Could you check a few things on this model? Use its own coordinates, in mm. Give positions to 0.01 mm unless a question says otherwise; leave off trailing zeros. Write each loop counter-clockwise with the first axis right and the second up, starting at its lowest first coordinate (ties: lowest second). Pieces come first, ordered by that corner, then holes. Notation, with made-up numbers: M 65.5,30.25 L 115.5,30.25 A14 cw 115.5,34.25 Z; hole C -3.5,69.25 d9. An arc over 180 degrees is marked long. One line per item, written item: value.
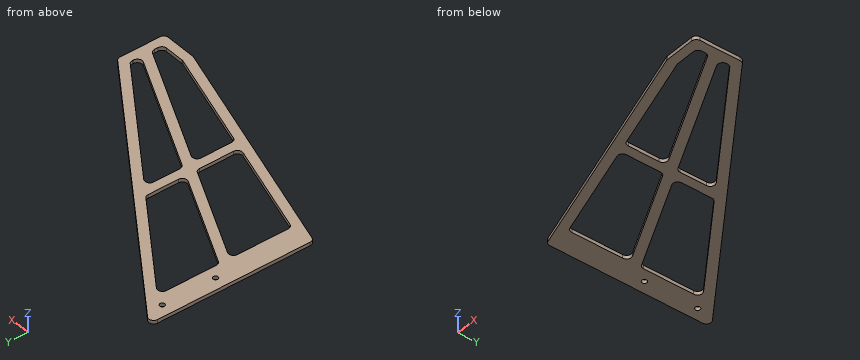
```python
from build123d import *

# Parameters (mm, degrees)
EXTRUDE_1_DEPTH     = 3
SKETCH_2_R          = 2.1
CUT_EXTRUDE_1_DEPTH = 39
CUT_EXTRUDE_2_DEPTH = 10
FILLET_1_R          = 4
FILLET_2_R          = 4


with BuildPart() as part:
    # Эскиз1 → Бобышка-Вытянуть1 (new body)
    with BuildSketch(Plane.XY):
        Polygon((0, 0), (0, 140), (230, -20), (230, -60), (200, -60), align=None)
    extrude(amount=EXTRUDE_1_DEPTH)

    # Эскиз2 → Вырез-Вытянуть1 (cut)
    with BuildSketch(Plane.XY.offset(3)):
        with Locations((10, 75)):
            Circle(SKETCH_2_R)
        with Locations((10, 120.2)):
            Circle(SKETCH_2_R)
    extrude(amount=-CUT_EXTRUDE_1_DEPTH, mode=Mode.SUBTRACT)

    # Эскиз5 → Вырез-Вытянуть2 (cut)
    with BuildSketch(Plane.XY.offset(3)):
        Polygon((222, -24.180122244), (222, -33.649029765), (114, 18.445995751), (114, 50.950312538), align=None)
        Polygon((20, 63.787962403), (106, 22.304886529), (106, 56.51552993), (20, 116.341616886), align=None)
        Polygon((20, 54.90589969), (106, 13.422823816), (106, -23.447754793), (20, 2.352245207), align=None)
        Polygon((201.17415069, -52), (222, -52), (222, -42.531092479), (114, 9.563933037), (114, -25.847754793), align=None)
    extrude(amount=-CUT_EXTRUDE_2_DEPTH, mode=Mode.SUBTRACT)

    # Скругление1
    fillet_1_edges = [part.edges().sort_by_distance(p)[0] for p in [
        (0, 0, 1.5),
        (0, 140, 1.5),
        (230, -20, 1.5),
        (230, -60, 1.5),
        (200, -60, 1.5),
    ]]
    fillet(fillet_1_edges, radius=FILLET_1_R)

    # Скругление2
    fillet_2_edges = [part.edges().sort_by_distance(p)[0] for p in [
        (20, 2.352245207, 1.5),
        (20, 54.90589969, 1.5),
        (106, 13.422823816, 1.5),
        (106, -23.447754793, 1.5),
        (114, 50.950312538, 1.5),
        (222, -24.180122244, 1.5),
        (222, -33.649029765, 1.5),
        (114, 18.445995751, 1.5),
        (222, -42.531092479, 1.5),
        (222, -52, 1.5),
        (201.17415069, -52, 1.5),
        (114, -25.847754793, 1.5),
        (114, 9.563933037, 1.5),
        (20, 116.341616886, 1.5),
        (106, 56.51552993, 1.5),
        (106, 22.304886529, 1.5),
        (20, 63.787962403, 1.5),
    ]]
    fillet(fillet_2_edges, radius=FILLET_2_R)


solid = part.part
```
1) I'm going to push flat-ended pins straight in: pin 1 (6 mm diameter, centred on x = 80, y = 87.5, fed in from -Z); pin 2 (1.5 mm diameter, centred on y = -8, z = 1, fed in from +X); pin 3 (1.5 mm diameter, centred on x = 212, z = 1.5, fed in from +Y); pin 4 (0.9 mm diameter, centred on y = 33, z = 1, fed in from +X). Where does each tip first touch, or does it pass through?
Outcome:
pin 1: stops at z = 0
pin 2: stops at x = 213.83
pin 3: stops at y = -6.96
pin 4: stops at x = 154.46
2) If we section it at B-B, the plane z = 2: Give the number of separate pieces and of enclosed holes in the cut face, then the cut area to 3 significant figures.
Outcome:
separate pieces: 1
enclosed holes: 6
area: 9,100 mm^2
3) If we section it at C-C, the plane x = 17.5: Write out the boundary of the cut face in (y, z).
Outcome:
outline: M -5.25,0 L 127.83,0 L 127.83,3 L -5.25,3 Z
4) Please list where these lines run through material, in increasing order: L1, parallel to Y at x = 43.5, z = 2.4; L2, parallel to X at y = 8, z = 1.2; L3, parallel to Y at x = 10, z = 1.2. Write a range as from..to.
Outcome:
L1: y = -13.05..-4.7, 43.57..52.45, 99.99..109.74
L2: x = 0..20, 106..135.66, 175.74..189.75
L3: y = -3..72.9, 77.1..118.1, 122.3..133.04
5) If we section it at A-A, the plane x = 85: Write out the boundary of the cut face in (y, z).
Outcome:
outline: M -25.5,0 L -17.15,0 L -17.15,3 L -25.5,3 Z; M 23.55,0 L 32.43,0 L 32.43,3 L 23.55,3 Z; M 71.12,0 L 80.87,0 L 80.87,3 L 71.12,3 Z
